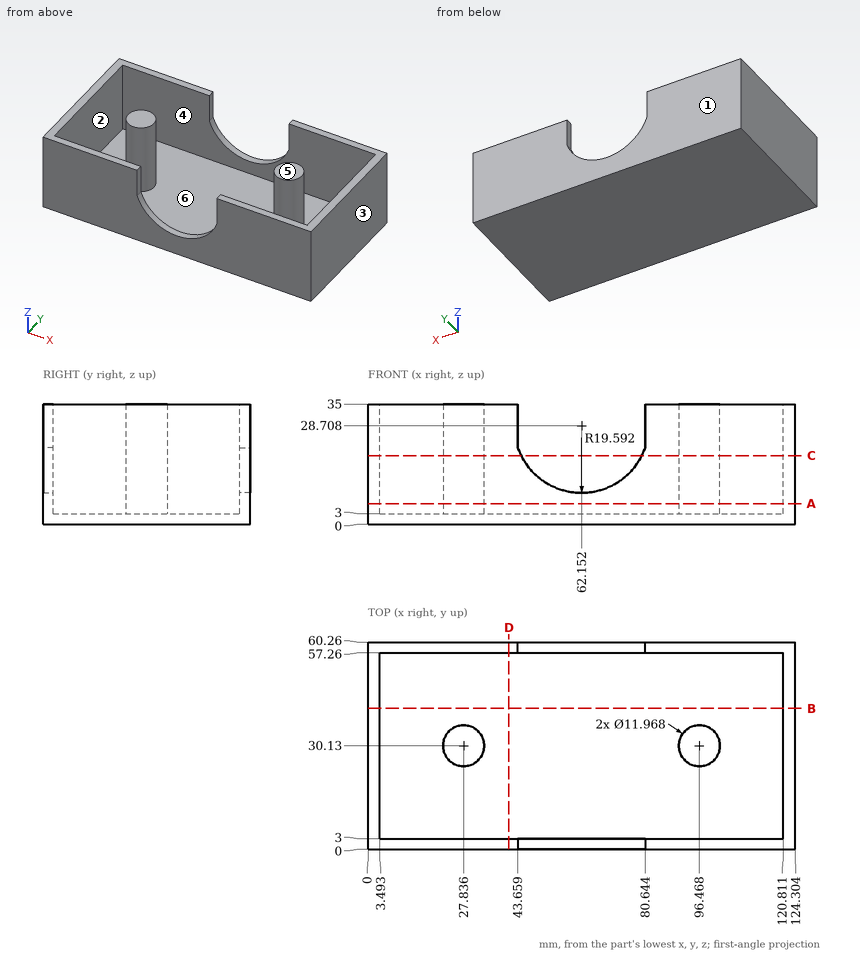
For this review, use the dimensioned drawing (mm, ordinates from the lowest corner) and the shaded views. A direction names the side the tool comes from. Round coordinates to 2 decimals unless told otherwise and drop trailing zeros. Order: outer loops, then holes, each group sorted by start corner. A loop starts at its lowest first (then second) coordinate and runs counter-clockwise, first axis right, second up. Notation, with made-up numbers: (81, -30) - (133, -30) arc R20 ccw to (133, -6) - close; hole circle Ø3 at (-7.75, 69). An arc over 180 degrees is marked (long way). Use one line per item in the form item = value.
Q1. Tool access review of the marked faces 5 and 6: name each direction out of +Z, -Z, +X, -X, +Y, -Y from which nothing blocks a thin tool from reaching the whole face with its end or side.
Response values:
face_5 = +Z, +X, -X, +Y, -Y
face_6 = +Z
Q2. Add section D-D on x = 41. Give the boundary of the cut face in (y, z).
Response values:
outline = (0, 0) - (60.26, 0) - (60.26, 35) - (57.26, 35) - (57.26, 3) - (3, 3) - (3, 35) - (0, 35) - close
Q3. Add section B-B on y = 41. Give the boundary of the cut face in (x, z).
Response values:
outline = (0, 0) - (124.3, 0) - (124.3, 35) - (120.81, 35) - (120.81, 3) - (3.49, 3) - (3.49, 35) - (0, 35) - close
Q4. To check wall thickness, follow line 1 (Y direction, x = 16, z = 15); line 2 (X direction, y = 30.5, z = 26.5) (1 decimal); line 3 (X direction, y = 16, z = 6.5). State the ranges of each line that lie inside material, in increasing order.
Response values:
line_1 = 0 to 3, 57.26 to 60.26
line_2 = 0 to 3.5, 21.9 to 33.8, 90.5 to 102.4, 120.8 to 124.3
line_3 = 0 to 3.49, 120.81 to 124.3
Q5. Add section C-C on z = 20. Give the boundary of the cut face in (x, y).
Response values:
outline = (0, 0) - (44.6, 0) - (44.6, 3) - (3.49, 3) - (3.49, 57.26) - (44.6, 57.26) - (44.6, 60.26) - (0, 60.26) - close; circle Ø11.97 at (27.84, 30.13); (79.7, 0) - (124.3, 0) - (124.3, 60.26) - (79.7, 60.26) - (79.7, 57.26) - (120.81, 57.26) - (120.81, 3) - (79.7, 3) - close; circle Ø11.97 at (96.47, 30.13)
Q6. Mouldability with a two-part tool opening along Y and no side actions: class the marked faces 1, 2, 3 and 4 as pulls with the +Y half, pulls with the -Y half, needs draft (parallel to the pull), parting line crosses it, or undercut.
Response values:
face_1 = pulls with the +Y half
face_2 = undercut
face_3 = needs draft
face_4 = undercut
Q7. Add section A-A on z = 6. Give the boundary of the cut face in (x, y).
Response values:
outline = (0, 0) - (124.3, 0) - (124.3, 60.26) - (0, 60.26) - close; circle Ø11.97 at (27.84, 30.13); circle Ø11.97 at (96.47, 30.13); hole (3.49, 3) - (120.81, 3) - (120.81, 57.26) - (3.49, 57.26) - close
Q8. Clearance check with flat-ended pins moving along their axes: P1, Ø1.5, axis at y = 43, z = 26, coming from the -X side; P2, Ø16.5, axis at x = 61, y = 20.5, coming from the +Z side. State where each tip first meets the part, or that it passes through.
Response values:
P1 = 0
P2 = 3
